The model under review builds one solid part; all positions refer to its coordinate system, in mm. A direction names the side the tool comes from. Round coordinates to 2 decimals unless told otherwise and drop trailing zeros. Loops run counter-clockwise (first coordinate to the right, second up) from the corner with the lowest first, then second, coordinate; pieces in that order, holes last. Notation, with made-up numbers: M 46.5,-8 L 95.5,-8 A31 cw 95.5,24 Z; hole C -10.75,43 d3. An arc over 180 degrees is marked long. Answer as a JSON object with one key per item and string values. Group by question number.
Item 1: Consider section C-C (y = -9.25). State how many separate pieces and enclosed holes the cut face has, and give its area (3 significant figures).
Item 2: To check wall thickness, follow line 1 (X direction, y = -13.25, z = 27.5); line 2 (X direction, y = -4.25, z = 30); line 3 (X direction, y = -25.25, z = -16.5). State the ranges of each line that lie inside material, in increasing order.
Item 3: Tool access review of faces 1 (the face through (23.9, -22.5, 29.3)), 2 (the face through (18.5, -12, 31)), 3 (the face through (1, -15, 35)): name each direction out of +Z, -Z, +X, -X, +Y, -Y from which nothing blocks a thin tool from reaching the whole face with its end or side.
Item 4: Consider section A-A (z = 12). Give the boundary of the cut face in (x, y).
Item 5: The part is to be moulded in two halves that separate along X. For faces 4 (the face through (-1, -15, -35)), 5 (the face through (-47, -22.5, -29)), 6 (the face through (54.1, -14.58, -34.14)), say which applies: +X half, -X half, draft (parallel to the pull), parting line (faces both ways), or undercut.
Item 6: Insertion check: P1, Ø9, axis at x = 44, z = -28, coming from the -Y side; P2, Ø3.5, axis at x = 25.5, z = 25.5, coming from the -Y side. Each pin has a flat end and moves straight along its axis. Give the tip position at first contact, or say it passes through.
Item 7: Consider section B-B (x = -37). Give the boundary of the cut face in (y, z).
```python
from build123d import *

# Parameters (mm, degrees)
BOSS_EXTRUDE1_DEPTH  = 2.5
BOSS_EXTRUDE6_DEPTH  = 24.5
CUT_EXTRUDE7_REACH   = 72.562
SKETCH3_R            = 2.5
BOSS_EXTRUDE11_START = -24.5
SKETCH12_R           = 1.5
BOSS_EXTRUDE11_DEPTH = 20
CUT_EXTRUDE11_REACH  = 120.55
SKETCH13_R           = 6.15
BOSS_EXTRUDE13_START = -4.5
SKETCH12_5_R         = 1.5
BOSS_EXTRUDE13_DEPTH = 2
CUT_EXTRUDE13_DEPTH  = 2.5


with BuildPart() as part:
    # Sketch1 → Boss-Extrude1 (new body)
    with BuildSketch(Plane(origin=(0, 0, 0), x_dir=(1, 0, 0), z_dir=(0, 1, 0))):
        with BuildLine():
            Line((-52, -35), (52, -35))
            ThreePointArc((52, -35), (54.121320344, -34.121320344), (55, -32))
            Line((55, -32), (55, 32))
            ThreePointArc((55, 32), (54.121320344, 34.121320344), (52, 35))
            Line((52, 35), (-52, 35))
            ThreePointArc((-52, 35), (-54.121320344, 34.121320344), (-55, 32))
            Line((-55, 32), (-55, -32))
            ThreePointArc((-55, -32), (-54.121320344, -34.121320344), (-52, -35))
        make_face()
    extrude(amount=-BOSS_EXTRUDE1_DEPTH)

    # Sketch7 → Boss-Extrude6 (add)
    with BuildSketch(Plane.XZ.offset(2.5)):
        with BuildLine():
            Line((-55, 32), (-55, -32))
            ThreePointArc((-55, -32), (-54.121320344, -34.121320344), (-52, -35))
            Line((-52, -35), (52, -35))
            ThreePointArc((52, -35), (54.121320344, -34.121320344), (55, -32))
            Line((55, -32), (55, 32))
            ThreePointArc((55, 32), (54.121320344, 34.121320344), (52, 35))
            Line((52, 35), (-52, 35))
            ThreePointArc((-52, 35), (-54.121320344, 34.121320344), (-55, 32))
        make_face()
        with BuildLine():
            Line((-53.5, 32), (-53.5, -32))
            ThreePointArc((-53.5, -32), (-53.060660172, -33.060660172), (-52, -33.5))
            Line((-52, -33.5), (52, -33.5))
            ThreePointArc((52, -33.5), (53.060660172, -33.060660172), (53.5, -32))
            Line((53.5, -32), (53.5, 32))
            ThreePointArc((53.5, 32), (53.060660172, 33.060660172), (52, 33.5))
            Line((52, 33.5), (-52, 33.5))
            ThreePointArc((-52, 33.5), (-53.060660172, 33.060660172), (-53.5, 32))
        make_face(mode=Mode.SUBTRACT)
    extrude(amount=BOSS_EXTRUDE6_DEPTH)

    # Sketch3 → Cut-Extrude7 (cut, up to next)
    with BuildSketch(Plane(origin=(0, 0, 0), x_dir=(1, 0, 0), z_dir=(0, 1, 0)), mode=Mode.PRIVATE) as cut_extrude7_sk1:
        with Locations(Location((-20.1, -27.5, 0), (0, 0, 270))):
            Circle(SKETCH3_R)
    cut_extrude7_tool1 = extrude(cut_extrude7_sk1.sketch, amount=-CUT_EXTRUDE7_REACH, mode=Mode.PRIVATE) & part.part
    # Sketch3 → Cut-Extrude7 (cut, up to next)
    with BuildSketch(Plane(origin=(0, 0, 0), x_dir=(1, 0, 0), z_dir=(0, 1, 0)), mode=Mode.PRIVATE) as cut_extrude7_sk2:
        with Locations(Location((-9.6, -27.5, 0), (0, 0, 270))):
            Circle(SKETCH3_R)
    cut_extrude7_tool2 = extrude(cut_extrude7_sk2.sketch, amount=-CUT_EXTRUDE7_REACH, mode=Mode.PRIVATE) & part.part
    # Sketch3 → Cut-Extrude7 (cut, up to next)
    with BuildSketch(Plane(origin=(0, 0, 0), x_dir=(1, 0, 0), z_dir=(0, 1, 0)), mode=Mode.PRIVATE) as cut_extrude7_sk3:
        with Locations(Location((0.5, -27.5, 0), (0, 0, 270))):
            Circle(SKETCH3_R)
    cut_extrude7_tool3 = extrude(cut_extrude7_sk3.sketch, amount=-CUT_EXTRUDE7_REACH, mode=Mode.PRIVATE) & part.part
    # Sketch3 → Cut-Extrude7 (cut, up to next)
    with BuildSketch(Plane(origin=(0, 0, 0), x_dir=(1, 0, 0), z_dir=(0, 1, 0)), mode=Mode.PRIVATE) as cut_extrude7_sk4:
        with Locations(Location((10.5, -27.5, 0), (0, 0, 270))):
            Circle(SKETCH3_R)
    cut_extrude7_tool4 = extrude(cut_extrude7_sk4.sketch, amount=-CUT_EXTRUDE7_REACH, mode=Mode.PRIVATE) & part.part
    add(cut_extrude7_tool1.solids().sort_by_distance((-20.1, 0, 27.5))[0], mode=Mode.SUBTRACT)
    add(cut_extrude7_tool2.solids().sort_by_distance((-9.6, 0, 27.5))[0], mode=Mode.SUBTRACT)
    add(cut_extrude7_tool3.solids().sort_by_distance((0.5, 0, 27.5))[0], mode=Mode.SUBTRACT)
    add(cut_extrude7_tool4.solids().sort_by_distance((10.5, 0, 27.5))[0], mode=Mode.SUBTRACT)

    # Sketch12 → Boss-Extrude11 (add)
    # profile 1 of 6: a face of its own
    with BuildSketch(Plane.XZ.offset(27).offset(BOSS_EXTRUDE11_START)):
        with BuildLine():
            Line((-39.5, 27.5), (-39.5, 33.5))
            Line((-39.5, 33.5), (-52, 33.5))
            ThreePointArc((-52, 33.5), (-53.060660172, 33.060660172), (-53.5, 32))
            Line((-53.5, 32), (-53.5, 22.5))
            Line((-53.5, 22.5), (-44.5, 22.5))
            ThreePointArc((-44.5, 22.5), (-40.964466094, 23.964466094), (-39.5, 27.5))
        make_face()
        with Locations(Location((-45.5, 27.5, 0), (0, 0, 270))):
            Circle(SKETCH12_R, mode=Mode.SUBTRACT)
    # profile 2 of 6: a face of its own
    with BuildSketch(Plane.XZ.offset(27).offset(BOSS_EXTRUDE11_START)):
        with BuildLine():
            Line((29.5, 33.5), (18.5, 33.5))
            Line((18.5, 33.5), (18.5, 27.5))
            ThreePointArc((18.5, 27.5), (19.964466094, 23.964466094), (23.5, 22.5))
            Line((23.5, 22.5), (24.5, 22.5))
            ThreePointArc((24.5, 22.5), (28.035533906, 23.964466094), (29.5, 27.5))
            Line((29.5, 27.5), (29.5, 33.5))
        make_face()
        with Locations(Location((24.5, 27.5, 0), (0, 0, 270))):
            Circle(SKETCH12_R, mode=Mode.SUBTRACT)
    # profile 3 of 6: a face of its own
    with BuildSketch(Plane.XZ.offset(27).offset(BOSS_EXTRUDE11_START)):
        with BuildLine():
            Line((18.5, -27.5), (18.5, -33.5))
            Line((18.5, -33.5), (29.5, -33.5))
            Line((29.5, -33.5), (29.5, -27.5))
            ThreePointArc((29.5, -27.5), (28.035533906, -23.964466094), (24.5, -22.5))
            Line((24.5, -22.5), (23.5, -22.5))
            ThreePointArc((23.5, -22.5), (19.964466094, -23.964466094), (18.5, -27.5))
        make_face()
        with Locations(Location((24.5, -27.5, 0), (0, 0, 270))):
            Circle(SKETCH12_R, mode=Mode.SUBTRACT)
    # profile 4 of 6: a face of its own
    with BuildSketch(Plane.XZ.offset(27).offset(BOSS_EXTRUDE11_START)):
        with BuildLine():
            Line((-44.5, -22.5), (-53.5, -22.5))
            Line((-53.5, -22.5), (-53.5, -32))
            ThreePointArc((-53.5, -32), (-53.060660172, -33.060660172), (-52, -33.5))
            Line((-52, -33.5), (-39.5, -33.5))
            Line((-39.5, -33.5), (-39.5, -27.5))
            ThreePointArc((-39.5, -27.5), (-40.964466094, -23.964466094), (-44.5, -22.5))
        make_face()
        with Locations(Location((-45.5, -27.5, 0), (0, 0, 270))):
            Circle(SKETCH12_R, mode=Mode.SUBTRACT)
    # profile 5 of 6: a face of its own
    with BuildSketch(Plane.XZ.offset(27).offset(BOSS_EXTRUDE11_START)):
        with BuildLine():
            Line((52, 33.5), (39.5, 33.5))
            Line((39.5, 33.5), (39.5, 27.5))
            ThreePointArc((39.5, 27.5), (40.964466094, 23.964466094), (44.5, 22.5))
            Line((44.5, 22.5), (53.5, 22.5))
            Line((53.5, 22.5), (53.5, 32))
            ThreePointArc((53.5, 32), (53.060660172, 33.060660172), (52, 33.5))
        make_face()
        with Locations(Location((45.5, 27.5, 0), (0, 0, 270))):
            Circle(SKETCH12_R, mode=Mode.SUBTRACT)
    # profile 6 of 6: a face of its own
    with BuildSketch(Plane.XZ.offset(27).offset(BOSS_EXTRUDE11_START)):
        with BuildLine():
            Line((53.5, -32), (53.5, -22.5))
            Line((53.5, -22.5), (44.5, -22.5))
            ThreePointArc((44.5, -22.5), (40.964466094, -23.964466094), (39.5, -27.5))
            Line((39.5, -27.5), (39.5, -33.5))
            Line((39.5, -33.5), (52, -33.5))
            ThreePointArc((52, -33.5), (53.060660172, -33.060660172), (53.5, -32))
        make_face()
        with Locations(Location((45.5, -27.5, 0), (0, 0, 270))):
            Circle(SKETCH12_R, mode=Mode.SUBTRACT)
    extrude(amount=BOSS_EXTRUDE11_DEPTH)

    # Sketch13 → Cut-Extrude11 (cut, up to next)
    with BuildSketch(Plane(origin=(55, 0, 0), x_dir=(0, 0, -1), z_dir=(1, 0, 0)), mode=Mode.PRIVATE) as cut_extrude11_sk1:
        with Locations((-12, -17)):
            Circle(SKETCH13_R)
    cut_extrude11_tool1 = extrude(cut_extrude11_sk1.sketch, amount=-CUT_EXTRUDE11_REACH, mode=Mode.PRIVATE) & part.part
    add(cut_extrude11_tool1.solids().sort_by_distance((55, -17, 12))[0], mode=Mode.SUBTRACT)

    # Sketch12<5> → Boss-Extrude13 (add)
    # profile 1 of 2: a face of its own
    with BuildSketch(Plane.XZ.offset(27).offset(BOSS_EXTRUDE13_START)):
        with BuildLine():
            Line((44.5, 22.5), (53.5, 22.5))
            Line((53.5, 22.5), (53.5, 32))
            ThreePointArc((53.5, 32), (53.060660172, 33.060660172), (52, 33.5))
            Line((52, 33.5), (39.5, 33.5))
            Line((39.5, 33.5), (39.5, 27.5))
            ThreePointArc((39.5, 27.5), (40.964466094, 23.964466094), (44.5, 22.5))
        make_face()
        with Locations(Location((45.5, 27.5, 0), (0, 0, 270))):
            Circle(SKETCH12_5_R, mode=Mode.SUBTRACT)
    # profile 2 of 2: a face of its own
    with BuildSketch(Plane.XZ.offset(27).offset(BOSS_EXTRUDE13_START)):
        with BuildLine():
            Line((39.5, -27.5), (39.5, -33.5))
            Line((39.5, -33.5), (52, -33.5))
            ThreePointArc((52, -33.5), (53.060660172, -33.060660172), (53.5, -32))
            Line((53.5, -32), (53.5, -22.5))
            Line((53.5, -22.5), (44.5, -22.5))
            ThreePointArc((44.5, -22.5), (40.964466094, -23.964466094), (39.5, -27.5))
        make_face()
        with Locations(Location((45.5, -27.5, 0), (0, 0, 270))):
            Circle(SKETCH12_5_R, mode=Mode.SUBTRACT)
    extrude(amount=BOSS_EXTRUDE13_DEPTH)

    # Sketch14 → Cut-Extrude13 (cut)
    with BuildSketch(Plane(origin=(0, 0, 0), x_dir=(1, 0, 0), z_dir=(0, 1, 0))):
        with BuildLine():
            Line((-52, -35), (52, -35))
            ThreePointArc((52, -35), (54.121320344, -34.121320344), (55, -32))
            Line((55, -32), (55, 32))
            ThreePointArc((55, 32), (54.121320344, 34.121320344), (52, 35))
            Line((52, 35), (-52, 35))
            ThreePointArc((-52, 35), (-54.121320344, 34.121320344), (-55, 32))
            Line((-55, 32), (-55, -32))
            ThreePointArc((-55, -32), (-54.121320344, -34.121320344), (-52, -35))
        make_face()
    extrude(amount=-CUT_EXTRUDE13_DEPTH, mode=Mode.SUBTRACT)


solid = part.part
```
Geometry results:
{
 "1": {"separate pieces": "1", "enclosed holes": "7", "area": "1,300 mm^2"},
 "2": {"line 1": "x = -55 to -47, -44 to -39.5, 18.5 to 23, 26 to 29.5, 39.5 to 44, 47 to 55", "line 2": "x = -55 to -39.5, 18.5 to 29.5, 39.5 to 55", "line 3": "x = -55 to -53.5, 53.5 to 55"},
 "3": {"face 1": "-Y", "face 2": "+Y, -Y", "face 3": "+Z, +X, -X, +Y, -Y"},
 "4": {"outline": "M -55,-27 L -53.5,-27 L -53.5,-2.5 L -55,-2.5 Z; M 53.5,-27 L 55,-27 L 55,-23.15 L 53.5,-23.15 Z; M 53.5,-10.85 L 55,-10.85 L 55,-2.5 L 53.5,-2.5 Z"},
 "5": {"face 4": "draft", "face 5": "undercut", "face 6": "+X half"},
 "6": {"P1": "stops at y = -24.5", "P2": "stops at y = -22.5"},
 "7": {"outline": "M -27,-35 L -2.5,-35 L -2.5,-33.5 L -27,-33.5 Z; M -27,33.5 L -2.5,33.5 L -2.5,35 L -27,35 Z"}
}
